from build123d import *

# Parameters (mm, degrees)
SKETCH1_R         = 12.5
EXTRUDE1_DEPTH    = 1.016
SKETCH2_R         = 12
SKETCH2_R_2       = 8.5
SKETCH2_R_3       = 8
SKETCH2_R_4       = 3
SKETCH2_R_5       = 2.5
EXTRUDE2_DEPTH    = 0.01
CIRPATTERN1_COUNT = 3
SKETCH6_R         = 2.0113
EXTRUDE5_DEPTH    = 0.01


with BuildPart() as part:
    # Sketch1 → Extrude1 (new body)
    with BuildSketch(Plane.XY):
        Circle(SKETCH1_R)
    extrude(amount=EXTRUDE1_DEPTH)

    # Sketch2 → Extrude2 (add)
    # profile 1 of 3: a face of its own
    with BuildSketch(Plane.XY.offset(1.016)):
        with Locations(Location((0, 0, 0), (0, 0, 180))):
            Circle(SKETCH2_R)
        with Locations(Location((0, 0, 0), (0, 0, 180))):
            Circle(SKETCH2_R_2, mode=Mode.SUBTRACT)
    # profile 2 of 3: a face of its own
    with BuildSketch(Plane.XY.offset(1.016)):
        with Locations(Location((0, 0, 0), (0, 0, 180))):
            Circle(SKETCH2_R_3)
        with Locations(Location((0, 0, 0), (0, 0, 180))):
            Circle(SKETCH2_R_4, mode=Mode.SUBTRACT)
    # profile 3 of 3: a face of its own
    with BuildSketch(Plane.XY.offset(1.016)):
        with Locations(Location((0, 0, 0), (0, 0, 180))):
            Circle(SKETCH2_R_5)
    extrude(amount=EXTRUDE2_DEPTH)

    # Sketch4 → CSK for #0 Flat Head Machine Screw1 (revolve, cut)
    with BuildSketch(Plane(origin=(0, 10, 1.026), x_dir=(0, -1, 0), z_dir=(1, 0, 0))):
        Polygon((0, 0), (0, 1.026), (0.80645, 1.026), (0.80645, 0.810837172), (1.5113, 0), align=None)
    csk_for_0_flat_head_machine_screw1 = revolve(axis=Axis((0, 10, 7.376), (0, 0, -1)), mode=Mode.SUBTRACT)

    # CirPattern1: CSK for #0 Flat Head Machine Screw1 ×3 about axis
    cirpattern1_axis = Axis((0, 0, 0), (0, 0, 1))
    for i in range(1, CIRPATTERN1_COUNT):
        add(csk_for_0_flat_head_machine_screw1.rotate(cirpattern1_axis, i * 360 / CIRPATTERN1_COUNT), mode=Mode.SUBTRACT)

    # Sketch6 → Extrude5 (cut)
    with BuildSketch(Plane.XY.offset(1.026)):
        with Locations((0, 10)):
            Circle(SKETCH6_R)
        with Locations((-8.660254038, -5)):
            Circle(SKETCH6_R)
        with Locations((8.660254038, -5)):
            Circle(SKETCH6_R)
    extrude(amount=-EXTRUDE5_DEPTH, mode=Mode.SUBTRACT)


solid = part.part
The listing builds one solid part. Answer for the finished solid, in the listing's coordinates (mm). Round coordinates to 2 decimals unless told otherwise and drop trailing zeros. Write each loop counter-clockwise with the first axis right and the second up, starting at its lowest first coordinate (ties: lowest second). Pieces come first, ordered by that corner, then holes. Notation, with made-up numbers: (46, -13.5) - (67, -13.5) arc R5 cw to (67, -7.5) - close; hole circle Ø10 at (-30.5, 83.5). An arc over 180 degrees is marked (long way). Use a Markdown table: item, result. Add a question column.
1. A flat-ended cylindrical pin translates along its axis: P1, Ø1, axis at x = -8.66, y = -5, coming from the +Z side. Find the tip coordinate at first contact, or state that the pin passes through.
2. Consider line 1 (Y direction, x = 0, z = 0.1); line 2 (X direction, y = 10, z = 0.1); line 3 (X direction, y = -5, z = 0.15). Determine where each line is inside the solid, lowest interval first.
3. The part is cut by section C-C (z = 0.6). Write down the section's boundary in (x, y).
Reported:
| question | item | result |
|---|---|---|
| 1 | P1 | through |
| 2 | line 1 | -12.5 to 9.19, 10.81 to 12.5 |
| 2 | line 2 | -7.5 to -0.81, 0.81 to 7.5 |
| 2 | line 3 | -11.46 to -9.47, -7.85 to 7.85, 9.47 to 11.46 |
| 3 | outline | circle Ø25 at (0, 0); hole circle Ø2.28 at (-8.66, -5); hole circle Ø2.28 at (0, 10); hole circle Ø2.28 at (8.66, -5) |
